For this review, take the finished solid that the model builds, in its own axes (mm). Round coordinates to 2 decimals unless told otherwise and drop trailing zeros. Write each loop counter-clockwise with the first axis right and the second up, starting at its lowest first coordinate (ties: lowest second). Pieces come first, ordered by that corner, then holes. Notation, with made-up numbers: (-27.5, 0) -> (5.5, 0) arc R27 cw to (5.5, 16) -> close; hole circle Ø2 at (83.5, 1.5). An arc over 180 degrees is marked (long way). Write each question's results on one line, items separated by ' | '. Start each with the question number.
Item 1: Add section C-C (y = -6.5). State the section outline as (x, z) points.
Item 2: To check wall thickness, follow line 1 along Y through (x, z) = (-35, 2.85); line 2 along Y through (x, z) = (24, 1.5); line 3 along X through (y, z) = (5.5, 1.4). State the ranges of each line that lie inside material, in increasing order.
Item 3: Add section B-B (z = 0.6). Count the separate pieces of the cut face and the enclosed holes in it, plus the area to 3 significant figures.
Item 4: Add section A-A (y = -15). State the section outline as (x, z) points.
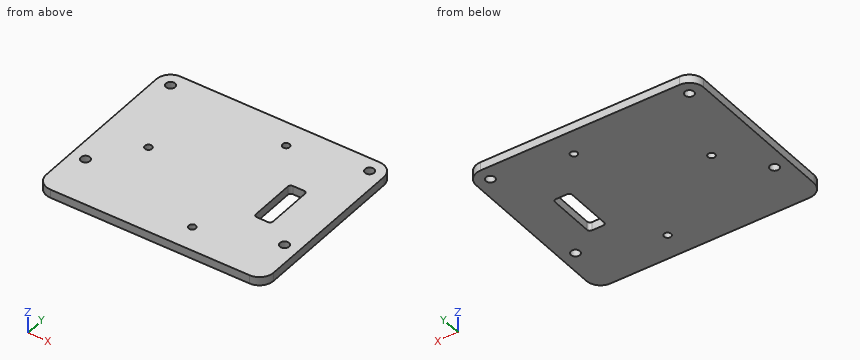
from build123d import *

# Parameters (mm, degrees)
SKETCH1_W           = 80
SKETCH1_H           = 65
SKETCH1_R           = 1.25
BOSS_EXTRUDE1_DEPTH = 3
FILLET1_R           = 5
SKETCH2_R           = 1.6
CUT_EXTRUDE1_DEPTH  = 52.626059311
SKETCH4_W           = 6
SKETCH4_H           = 18
CUT_EXTRUDE2_DEPTH  = 52.626059311
FILLET2_R           = 1


with BuildPart() as part:
    # Sketch1 → Boss-Extrude1 (new body)
    with BuildSketch(Plane.XY):
        Rectangle(SKETCH1_W, SKETCH1_H)
        with Locations((8.526833703, 23.400005474)):
            Circle(SKETCH1_R, mode=Mode.SUBTRACT)
        with Locations((8.526833703, -23.399994526)):
            Circle(SKETCH1_R, mode=Mode.SUBTRACT)
        with Locations((-23.393166297, 5.474e-06)):
            Circle(SKETCH1_R, mode=Mode.SUBTRACT)
    extrude(amount=BOSS_EXTRUDE1_DEPTH)

    # Fillet1
    fillet1_edges = [part.edges().sort_by_distance(p)[0] for p in [
        (-40, 32.5, 1.5),
        (40, 32.5, 1.5),
        (40, -32.5, 1.5),
        (-40, -32.5, 1.5),
    ]]
    fillet(fillet1_edges, radius=FILLET1_R)

    # Sketch2 → Cut-Extrude1 (cut, through all)
    with BuildSketch(Plane(origin=(0, 0, 0), x_dir=(-1, 0, 0), z_dir=(0, 0, -1))):
        with Locations((-35, 27.5)):
            Circle(SKETCH2_R)
        with Locations((-35, -15)):
            Circle(SKETCH2_R)
        with Locations((35, 27.5)):
            Circle(SKETCH2_R)
        with Locations((35, -15)):
            Circle(SKETCH2_R)
    extrude(amount=-CUT_EXTRUDE1_DEPTH, mode=Mode.SUBTRACT)

    # Sketch4 → Cut-Extrude2 (cut, through all)
    with BuildSketch(Plane(origin=(0, 0, 0), x_dir=(-1, 0, 0), z_dir=(0, 0, -1))):
        with Locations((-23, 0)):
            Rectangle(SKETCH4_W, SKETCH4_H)
    extrude(amount=-CUT_EXTRUDE2_DEPTH, mode=Mode.SUBTRACT)

    # Fillet2
    fillet2_edges = [part.edges().sort_by_distance(p)[0] for p in [
        (26, -9, 1.5),
        (26, 9, 1.5),
        (20, 9, 1.5),
        (20, -9, 1.5),
    ]]
    fillet(fillet2_edges, radius=FILLET2_R)


solid = part.part
Responses:
1) outline: (-40, 0) -> (20, 0) -> (20, 3) -> (-40, 3) -> close; (26, 0) -> (40, 0) -> (40, 3) -> (26, 3) -> close
2) line 1: y = -32.5 to -16.6, -13.4 to 25.9, 29.1 to 32.5 | line 2: y = -32.5 to -9, 9 to 32.5 | line 3: x = -40 to 20, 26 to 40
3) separate pieces: 1 | enclosed holes: 8 | area: 5,020 mm^2
4) outline: (-40, 0) -> (-36.6, 0) -> (-36.6, 3) -> (-40, 3) -> close; (-33.4, 0) -> (33.4, 0) -> (33.4, 3) -> (-33.4, 3) -> close; (36.6, 0) -> (40, 0) -> (40, 3) -> (36.6, 3) -> close
